Input: part model. Units: mm. Frame: model coordinates. Face numbers are marked on the shaded views. Coordinates: 2 decimals unless noted, no trailing zeros. Write each loop counter-clockwise with the first axis right and the second up, starting at its lowest first coordinate (ties: lowest second). Pieces come first, ordered by that corner, then holes.
1) Pin query (flat end, axial travel): pin 1 Ø1 at (y, z) = (6.5, -2) entering from -X; pin 2 Ø1.5 at (x, z) = (9.5, 7) entering from -Y; pin 3 Ø4 at (y, z) = (4.5, -10) entering from +X; pin 4 Ø7 at (x, z) = (0, 0) entering from +Y. Return the tip coordinate at first contact, or that it passes through.
2) Section query D-D (z = -5). Output: boundary loops of the cut face in (x, y).
3) Section query B-B (z = 0). Output: boundary loops of the cut face in (x, y).
4) Draft query along X for the marked faces 1, 2 and 3. Return one class per face: pulls with the +X half, pulls with the -X half, needs draft (parallel to the pull), parting line crosses it, or undercut.
5) Line query: L1, parallel to Z at x = 0, y = 3.5; L2, parallel to X at y = 4.5, z = 3; L3, parallel to Y at x = 12, z = 6.25. Output: solid intervals per line, ascending.
6) Section query C-C (y = 13). Output: boundary loops of the cut face in (x, z), then the cut area to 3 significant figures.
7) Section query A-A (x = 0). Output: boundary loops of the cut face in (y, z).
from build123d import *

# Parameters (mm, degrees)
F1_DEPTH = 12.7
F2_R     = 3.81
F3_DEPTH = 14.2885


with BuildPart() as f1:
    # F0 (on Top) → F1 (new body, symmetric)
    with BuildSketch(Plane.XY):
        Polygon((-19.05, 14.2875), (-4.7625, 0), (4.7625, 0), (19.05, 14.2875), align=None)
    extrude(amount=F1_DEPTH, both=True)

    # F2 (on Front) → F3 (cut, through all)
    with BuildSketch(Plane.XZ):
        Circle(F2_R)
    extrude(amount=-F3_DEPTH, mode=Mode.SUBTRACT)


solid = f1.part
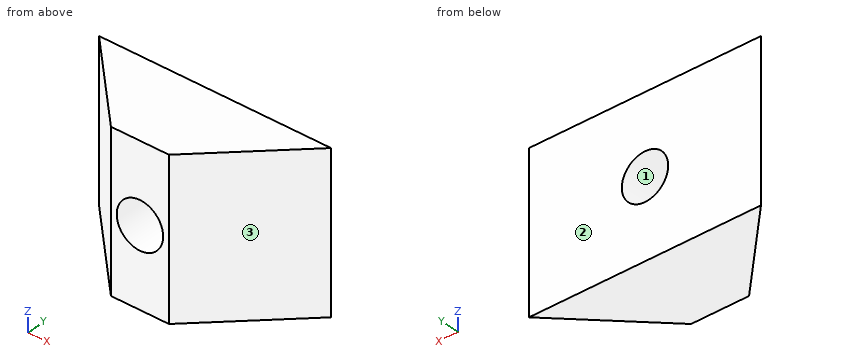
Answer:
1. pin 1: stops at x = -11.76
1. pin 2: stops at y = 3.99
1. pin 3: stops at x = 11.26
1. pin 4: passes through
2. outline: (-19.05, 14.29) - (-4.76, 0) - (4.76, 0) - (19.05, 14.29) - close
3. outline: (-19.05, 14.29) - (-4.76, 0) - (-3.81, 0) - (-3.81, 14.29) - close; (3.81, 0) - (4.76, 0) - (19.05, 14.29) - (3.81, 14.29) - close
4. face 1: undercut
4. face 2: needs draft
4. face 3: pulls with the +X half
5. L1: z = -12.7 to -3.81, 3.81 to 12.7
5. L2: x = -9.26 to -2.35, 2.35 to 9.26
5. L3: y = 7.24 to 14.29
6. outline: (-17.76, -12.7) - (17.76, -12.7) - (17.76, 12.7) - (-17.76, 12.7) - close; hole circle Ø7.62 at (0, 0)
6. area: 857 mm2
7. outline: (0, -12.7) - (14.29, -12.7) - (14.29, -3.81) - (0, -3.81) - close; (0, 3.81) - (14.29, 3.81) - (14.29, 12.7) - (0, 12.7) - close
